from build123d import *

# Parameters (mm, degrees)
BOSS_EXTRUDE5_DEPTH = 15
BOSS_EXTRUDE6_DEPTH = 10
BOSS_EXTRUDE7_DEPTH = 5
BOSS_EXTRUDE8_DEPTH = 15


with BuildPart() as part:
    # Sketch1_6 → Boss-Extrude5 (new body)
    with BuildSketch(Plane(origin=(0, 0, 0), x_dir=(1, 0, 0), z_dir=(0, 1, 0))):
        with BuildLine():
            ThreePointArc((103.929018633, 0), (98.929018633, 5), (93.929018633, 0))
            Line((93.929018633, 0), (103.929018633, 0))
        make_face()
        with BuildLine():
            Line((103.929018633, 0), (93.929018633, 0))
            ThreePointArc((93.929018633, 0), (98.929018633, -5), (103.929018633, 0))
        make_face()
    extrude(amount=BOSS_EXTRUDE5_DEPTH)

    # Sketch1_7 → Boss-Extrude6 (add)
    with BuildSketch(Plane(origin=(0, 0, 0), x_dir=(1, 0, 0), z_dir=(0, 1, 0))):
        with BuildLine():
            ThreePointArc((106.429018633, 0), (98.929018633, 7.5), (91.429018633, 0))
            Line((91.429018633, 0), (93.929018633, 0))
            ThreePointArc((93.929018633, 0), (98.929018633, 5), (103.929018633, 0))
            Line((103.929018633, 0), (106.429018633, 0))
        make_face()
        with BuildLine():
            Line((93.929018633, 0), (91.429018633, 0))
            ThreePointArc((91.429018633, 0), (98.929018633, -7.5), (106.429018633, 0))
            Line((106.429018633, 0), (103.929018633, 0))
            ThreePointArc((103.929018633, 0), (98.929018633, -5), (93.929018633, 0))
        make_face()
    extrude(amount=BOSS_EXTRUDE6_DEPTH)

    # Sketch1_8 → Boss-Extrude7 (add)
    with BuildSketch(Plane(origin=(0, 0, 0), x_dir=(1, 0, 0), z_dir=(0, 1, 0))):
        with BuildLine():
            ThreePointArc((106.429018633, 0), (98.929018633, -7.5), (91.429018633, 0))
            Line((91.429018633, 0), (91.429018633, -15))
            Line((91.429018633, -15), (106.429018633, -15))
            Line((106.429018633, -15), (106.429018633, 0))
        make_face()
    extrude(amount=BOSS_EXTRUDE7_DEPTH)

    # Sketch1_9 → Boss-Extrude8 (add)
    with BuildSketch(Plane(origin=(0, 0, 0), x_dir=(1, 0, 0), z_dir=(0, 1, 0))):
        Polygon((106.429018633, -15), (91.429018633, -15), (89.429018633, -15), (89.429018633, -30.12715853), (87.321654073, -55), (106.429018633, -30.12715853), (108.429018633, -15), align=None)
    extrude(amount=BOSS_EXTRUDE8_DEPTH)


solid = part.part
Design review of the part built by this model. Coordinates are the model's own, in mm. A direction names the side the tool comes from. Coordinates: 2 decimals unless noted, no trailing zeros. Loops run counter-clockwise (first coordinate to the right, second up) from the corner with the lowest first, then second, coordinate; pieces in that order, holes last. Notation, with made-up numbers: (-20.5, -33.5) -> (-9.5, -33.5) arc R23 ccw to (-9.5, -15.5) -> close; hole circle Ø3 at (57, 83.25). An arc over 180 degrees is marked (long way). Use a Markdown table: item, result. Add a question column.
Item 1: We need section C-C, the plane z = 46.5. Write out the cut boundary in (x, y), and give its area (3 significant figures).
Item 2: Wall thickness on L1, parallel to Y at x = 100.5, z = -5; L2, parallel to Z at x = 98.25, y = 14.25; L3, parallel to Z at x = 104, y = 9: over which ranges is each line inside the solid? List them lowest first. Write a range as from..to.
Item 3: Clearance check with flat-ended pins moving along their axes: P1, Ø1, axis at x = 104.5, z = 3.5, coming from the +Y side; P2, Ø2, axis at y = 3.5, z = 47, coming from the -X side; P3, Ø5, axis at x = 104, y = 8.5, coming from the -Z side. State where each tip first meets the part, or that it passes through.
Item 4: We need section A-A, the plane x = 96.25. Write out the cut boundary in (y, z).
Item 5: The part is to be moulded in two halves that separate along Z. For faces 4 (the flat face through (106.429, 2, 8)), 5 (the flat face through (104, 10, 2)), 6 (the flat face through (88.39, 7.4, 42.39)), 7 (the flat face through (96.74, 7.4, 42.74)), say which applies: +Z half, -Z half, draft (parallel to the pull), parting line (faces both ways), or undercut.
Item 6: We need section B-B, the plane z = 9. Write out the cut boundary in (x, y), and give its area (3 significant figures).
Item 7: Machinability: for faces 1 (the flat face through (99, 5, 11)), 2 (the flat face through (98, 0, 16)), 3 (the flat face through (91.429, 2, 7)), which of the approach directions +Z, -Z, +X, -X, +Y, -Y give a long, thin tool a straight path to every point of the face, cutting with its end or side? Answer none if there is none.
Numbers:
| question | item | result |
|---|---|---|
| 1 | outline | (88.04, 0) -> (93.85, 0) -> (93.85, 15) -> (88.04, 15) -> close |
| 1 | area | 87.1 mm^2 |
| 2 | L1 | y = 0..10 |
| 2 | L2 | z = -4.95..4.95, 15..40.77 |
| 2 | L3 | z = -5.53..5.53, 15..33.29 |
| 3 | P1 | stops at y = 10 |
| 3 | P2 | stops at x = 87.91 |
| 3 | P3 | stops at z = -7.05 |
| 4 | outline | (0, -7.01) -> (10, -7.01) -> (10, -4.22) -> (15, -4.22) -> (15, 4.22) -> (10, 4.22) -> (10, 7.01) -> (5, 7.01) -> (5, 15) -> (15, 15) -> (15, 43.38) -> (0, 43.38) -> close |
| 5 | face 4 | draft |
| 5 | face 5 | undercut |
| 5 | face 6 | -Z half |
| 5 | face 7 | +Z half |
| 6 | outline | (91.43, 0) -> (106.43, 0) -> (106.43, 5) -> (91.43, 5) -> close |
| 6 | area | 75.0 mm^2 |
| 7 | face 1 | +Y |
| 7 | face 2 | +Z, -Z, +X, -X, -Y |
| 7 | face 3 | -Z, -X, +Y, -Y |
